```python
from build123d import *

# Parameters (mm, degrees)
F1_DEPTH  = 12
F3_DEPTH  = 22.001
F5_DEPTH  = 3
F6_W      = 1.5
F6_H      = 12
F7_DEPTH  = 1
F8_W      = 1.5
F8_H      = 12
F9_DEPTH  = 1
F10_R     = 2.75
F11_DEPTH = 1.5
F12_R     = 2.25
F13_DEPTH = 25


with BuildPart() as f1:
    # F0 (on Front) → F1 (new body)
    with BuildSketch(Plane.XZ):
        with BuildLine():
            ThreePointArc((-9.5, 6.1146484713), (0, 10.6146484713), (9.5, 6.1146484713))
            Line((9.5, 6.1146484713), (11, 6.1146484713))
            Line((11, 6.1146484713), (11, 21.1146484713))
            Line((11, 21.1146484713), (-11, 21.1146484713))
            Line((-11, 21.1146484713), (-11, 6.1146484713))
            Line((-11, 6.1146484713), (-9.5, 6.1146484713))
        make_face()
    extrude(amount=F1_DEPTH)

    # F2 (on face) → F3 (cut, through all)
    with BuildSketch(Plane.YZ.offset(11)):
        Polygon((-12, 21.1146484713), (-12, 13.851130248), (-2.1519224699, 12.1146484713), (-0.75, 20.0653458872), (0, 20.0653458872), (0, 21.1146484713), align=None)
    extrude(amount=-F3_DEPTH, mode=Mode.SUBTRACT)

    # F4 (on face) → F5 (cut)
    with BuildSketch(Plane(origin=(-11, 0, 0), x_dir=(0, -1, 0), z_dir=(-1, 0, 0))):
        Polygon((0.75, 20.0653458872), (0, 20.0653458872), (0, 15.1146484713), (1.6229415278, 15.1146484713), align=None)
    extrude(amount=-F5_DEPTH, mode=Mode.SUBTRACT)

    # F6 (on face) → F7 (join)
    with BuildSketch(Plane(origin=(0, 0, 6.1146484713), x_dir=(1, 0, 0), z_dir=(0, 0, -1))):
        with Locations((-10.25, 6)):
            Rectangle(F6_W, F6_H)
    extrude(amount=F7_DEPTH)

    # F8 (on face) → F9 (join)
    with BuildSketch(Plane(origin=(0, 0, 6.1146484713), x_dir=(1, 0, 0), z_dir=(0, 0, -1))):
        with Locations((10.25, 6)):
            Rectangle(F8_W, F8_H)
    extrude(amount=F9_DEPTH)

    # F10 (on face) → F11 (cut)
    with BuildSketch(Plane(origin=(0, 2.006838501, 11.3813467058), x_dir=(1, 0, 0), z_dir=(0, 0.1736481777, 0.984807753))):
        with Locations((0, -8)):
            Circle(F10_R)
    extrude(amount=-F11_DEPTH, mode=Mode.SUBTRACT)

    # F12 (on face) → F13 (cut)
    with BuildSketch(Plane(origin=(0, 1.7463662345, 9.9041350763), x_dir=(1, 0, 0), z_dir=(0, 0.1736481777, 0.984807753))):
        with Locations((0, -8)):
            Circle(F12_R)
    extrude(amount=-F13_DEPTH, mode=Mode.SUBTRACT)


solid = f1.part
```
Source: CAD feature listing. Evaluate the final solid. Frame: model axes, mm. A direction names the side the tool comes from. Give positions to 0.01 mm unless a question says otherwise; leave off trailing zeros. Order: outer loops, then holes, each group sorted by start corner. A loop starts at its lowest first (then second) coordinate and runs counter-clockwise, first axis right, second up. Notation, with made-up numbers: (-24.75, -4.5) -> (13.25, -4.5) arc R11 cw to (13.25, 13.5) -> close; hole circle Ø1 at (72.5, 44.5). An arc over 180 degrees is marked (long way). Use a Markdown table: item, result.
Q1. Section B-B (z = 7.25). Return the cut outline in (x, y), and give its area (3 significant figures).
A:
| item | result |
|---|---|
| outline | (-11, -12) -> (-8.44, -12) -> (-8.44, 0) -> (-11, 0) -> close; (8.44, -12) -> (11, -12) -> (11, 0) -> (8.44, 0) -> close |
| area | 61.3 mm^2 |
Q2. First-contact query: P1, Ø3, axis at x = -1, y = -10.5, coming from the +Z side; P2, Ø1.3, axis at y = -1, z = 18, coming from the -X side; P3, Ø4, axis at x = 0, y = -1.5, coming from the -Z side. Flat tips, straight axial feed; report the tip coordinate or a pass-through.
A:
| item | result |
|---|---|
| P1 | z = 13.85 |
| P2 | x = -8 |
| P3 | z = 10.45 |
Q3. Section A-A (x = 0.5). Return the cut outline in (y, z).
A:
| item | result |
|---|---|
| outline | (-12, 10.6) -> (-8.48, 10.6) -> (-8.29, 11.67) -> (-8.8, 11.76) -> (-8.53, 13.24) -> (-12, 13.85) -> close; (-4.03, 10.6) -> (0, 10.6) -> (0, 20.07) -> (-0.75, 20.07) -> (-2.15, 12.11) -> (-3.21, 12.3) -> (-3.47, 10.82) -> (-3.97, 10.91) -> close |
Q4. Access query for faces 1 (the face through (0.15, -9.33, 13.38)), 2 (the face through (-9.5, -5.9, 5.6)), 3 (the face through (-0.488, -8.367, 11.266)), 4 (the face through (11, -6, 9)), 5 (the face through (-8, -1, 17)). Directions: +Z, -Z, +X, -X, +Y, -Y. A direction counts if a zero-diameter tool reaches every point of the face in a straight line with its end or side. Return the directions, or none.
A:
| item | result |
|---|---|
| face 1 | +Z, +X, -X |
| face 2 | -Z, +Y, -Y |
| face 3 | none |
| face 4 | +Z, -Z, +X, +Y, -Y |
| face 5 | +Z, -X, +Y, -Y |
Q5. Material intervals for line 1 (X direction, y = -1, z = 6); line 2 (X direction, y = -4.75, z = 11.25); line 3 (Z direction, x = 0, y = -2.25), sorted ascending. Write a range as [from, to].
A:
| item | result |
|---|---|
| line 1 | [-11, -9.5], [9.5, 11] |
| line 2 | [-11, -2.39], [2.39, 11] |
| line 3 | [10.61, 12.13] |
Q6. Pull-direction query (Z, two-part tool) for faces 6 (the face through (-11, -6, 9)), 7 (the face through (0.15, -1.46, 16.03)), 8 (the face through (-2.547, -5.916, 10.347)), 9 (the face through (-0.596, -8.644, 12.508)); classes: +Z half, -Z half, draft (parallel to the pull), parting line (faces both ways), or undercut.
A:
| item | result |
|---|---|
| face 6 | draft |
| face 7 | +Z half |
| face 8 | -Z half |
| face 9 | undercut |
Q7. Section C-C (y = -10). Return the cut outline in (x, z).
A:
| item | result |
|---|---|
| outline | (-11, 5.11) -> (-9.5, 5.11) -> (-9.5, 6.11) arc R12.28 cw to (9.5, 6.11) -> (9.5, 5.11) -> (11, 5.11) -> (11, 13.5) -> (-11, 13.5) -> close |
Q8. Section D-D (x = 7). Return the cut outline in (y, z).
A:
| item | result |
|---|---|
| outline | (-12, 8.42) -> (0, 8.42) -> (0, 20.07) -> (-0.75, 20.07) -> (-2.15, 12.11) -> (-12, 13.85) -> close |
